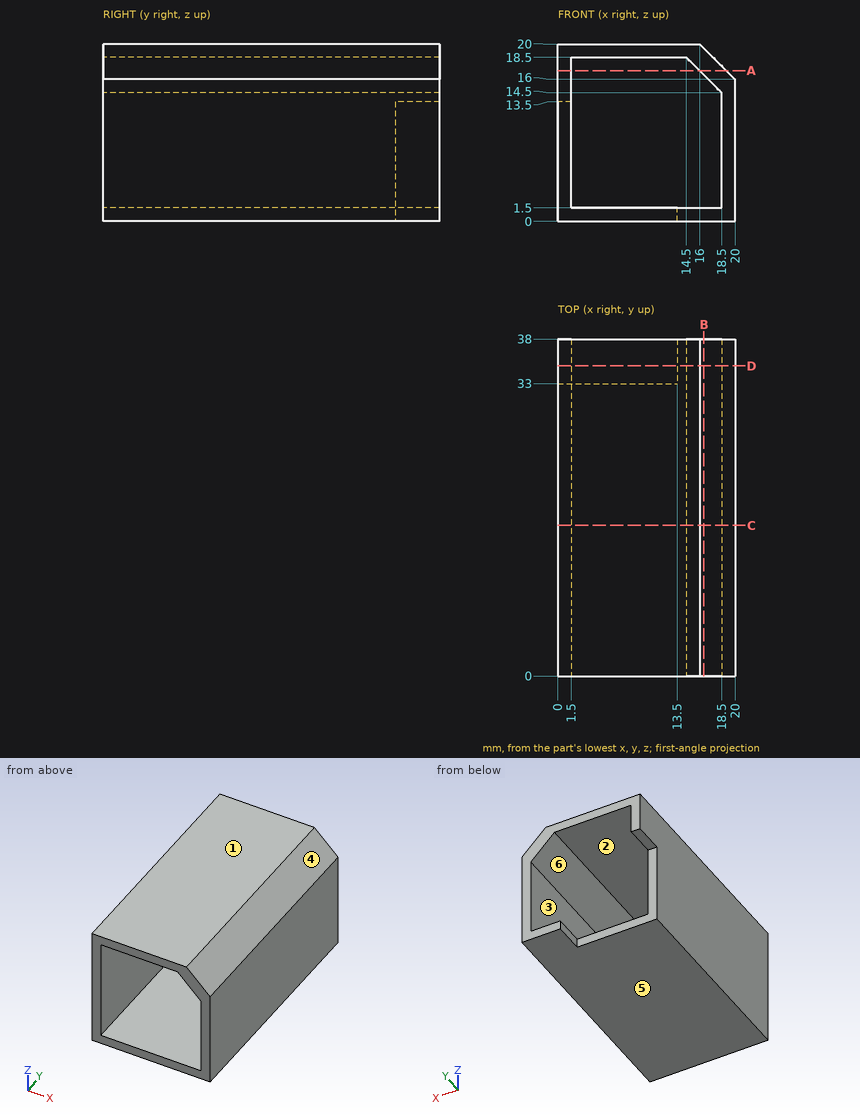
Design review of the part shown in the three views and the two pictorial views. Dimensions are in mm from the part's minimum x, y and z. A direction names the side the tool comes from. Coordinates: 2 decimals unless noted, no trailing zeros. Loops run counter-clockwise (first coordinate to the right, second up) from the corner with the lowest first, then second, coordinate; pieces in that order, holes last. Notation, with made-up numbers: (45, 88) - (65, 88) arc R21 ccw to (65, 107) - close; hole circle Ø3 at (22.5, 29). An arc over 180 degrees is marked (long way). Use a Markdown table: item, result. Add a question column.
Item 1: We need section B-B (x = 16.5). Give the boundary of the cut face in (y, z).
Item 2: For line 1 (X direction, y = 5, z = 14); line 2 (Z direction, x = 14.75, y = 14.5), list the stretches that pass through material, from the lowest coordinate up.
Item 3: We need section D-D (y = 35). Give the boundary of the cut face in (x, z), and give its area (4 significant figures).
Item 4: Mouldability with a two-part tool opening along X and no side actions: class the marked faces 1, 2, 3 and 4 as pulls with the +X half, pulls with the -X half, needs draft (parallel to the pull), parting line crosses it, or undercut.
Item 5: Tool access review of the marked faces 5 and 6: name each direction out of +Z, -Z, +X, -X, +Y, -Y from which nothing blocks a thin tool from reaching the whole face with its end or side.
Item 6: We need section A-A (z = 17). Give the boundary of the cut face in (x, y), and give its area (3 significant figures).
Item 7: Insertion check: pin 1 Ø11 at (x, z) = (7.5, 5.5) entering from +Y; pin 2 Ø1.6 at (x, y) = (1, 34.5) entering from -Z; pin 3 Ø0.8 at (y, z) = (36, 1) entering from -X. Each pin has a flat end and moves straight along its axis. Give the tip position at first contact, or say it passes through.
Item 8: We need section C-C (y = 17). Give the boundary of the cut face in (x, z).
Results list:
| question | item | result |
|---|---|---|
| 1 | outline | (0, 0) - (38, 0) - (38, 1.5) - (0, 1.5) - close; (0, 16.5) - (38, 16.5) - (38, 19.5) - (0, 19.5) - close |
| 2 | line 1 | x = 0 to 1.5, 18.5 to 20 |
| 2 | line 2 | z = 0 to 1.5, 18.25 to 20 |
| 3 | outline | (0, 13.5) - (1.5, 13.5) - (1.5, 18.5) - (14.5, 18.5) - (18.5, 14.5) - (18.5, 1.5) - (13.5, 1.5) - (13.5, 0) - (20, 0) - (20, 16) - (16, 20) - (0, 20) - close |
| 3 | area | 72.75 mm^2 |
| 4 | face 1 | needs draft |
| 4 | face 2 | undercut |
| 4 | face 3 | undercut |
| 4 | face 4 | pulls with the +X half |
| 5 | face 5 | -Z, +X, -X, +Y, -Y |
| 5 | face 6 | +Y, -Y |
| 6 | outline | (0, 0) - (1.5, 0) - (1.5, 38) - (0, 38) - close; (16, 0) - (19, 0) - (19, 38) - (16, 38) - close |
| 6 | area | 171 mm^2 |
| 7 | pin 1 | stops at y = 33 |
| 7 | pin 2 | stops at z = 13.5 |
| 7 | pin 3 | stops at x = 13.5 |
| 8 | outline | (0, 0) - (20, 0) - (20, 16) - (16, 20) - (0, 20) - close; hole (1.5, 1.5) - (18.5, 1.5) - (18.5, 14.5) - (14.5, 18.5) - (1.5, 18.5) - close |
